Design review of the part built by this model. Coordinates are the model's own, in mm. A direction names the side the tool comes from. Coordinates: 2 decimals unless noted, no trailing zeros. Write each loop counter-clockwise with the first axis right and the second up, starting at its lowest first coordinate (ties: lowest second). Pieces come first, ordered by that corner, then holes. Notation, with made-up numbers: (-33, 30) -> (-28, 30) arc R19 ccw to (-28, 44) -> close; hole circle Ø6 at (15, 76.5). An arc over 180 degrees is marked (long way). Write item = value, one per line. Start each with the question number.
```python
from build123d import *

# Parameters (mm, degrees)
SCHIZZO1_R                     = 3.5
SCHIZZO1_R_2                   = 1.75
ESTRUSIONE_ESTRUSIONE1_DEPTH   = 25
ESTRUSIONE_ESTRUSIONE1_2_DEPTH = 25
ESTRUSIONE_ESTRUSIONE1_3_DEPTH = 25
ESTRUSIONE_ESTRUSIONE1_4_DEPTH = 25
SCHIZZO1_3_R                   = 10.9
SCHIZZO1_3_R_2                 = 5
SCHIZZO1_3_R_3                 = 3
ESTRUSIONE_ESTRUSIONE2_DEPTH   = 3
ESTRUSIONE_ESTRUSIONE4_START   = 3
SCHIZZO1_5_R                   = 10.9
SCHIZZO1_5_R_2                 = 5
ESTRUSIONE_ESTRUSIONE4_DEPTH   = 3
RACCORDO1_R                    = 10


with BuildPart() as part:
    # Schizzo1 → Estrusione-Estrusione1 (new body)
    with BuildSketch(Plane(origin=(0, 0, 0), x_dir=(1, 0, 0), z_dir=(0, 1, 0))):
        with Locations(Location((-15.5, -15.5, 0), (0, 0, 270))):
            Circle(SCHIZZO1_R)
        with Locations(Location((-15.5, -15.5, 0), (0, 0, 270))):
            Circle(SCHIZZO1_R_2, mode=Mode.SUBTRACT)
    extrude(amount=ESTRUSIONE_ESTRUSIONE1_DEPTH)



with BuildPart() as body_2:
    # Schizzo1 → Estrusione-Estrusione1 2 (new body)
    with BuildSketch(Plane(origin=(0, 0, 0), x_dir=(1, 0, 0), z_dir=(0, 1, 0))):
        with Locations(Location((-15.5, 15.5, 0), (0, 0, 270))):
            Circle(SCHIZZO1_R)
        with Locations(Location((-15.5, 15.5, 0), (0, 0, 270))):
            Circle(SCHIZZO1_R_2, mode=Mode.SUBTRACT)
    extrude(amount=ESTRUSIONE_ESTRUSIONE1_2_DEPTH)


with BuildPart() as body_3:
    # Schizzo1 → Estrusione-Estrusione1 3 (new body)
    with BuildSketch(Plane(origin=(0, 0, 0), x_dir=(1, 0, 0), z_dir=(0, 1, 0))):
        with Locations(Location((15.5, 15.5, 0), (0, 0, 270))):
            Circle(SCHIZZO1_R)
        with Locations(Location((15.5, 15.5, 0), (0, 0, 270))):
            Circle(SCHIZZO1_R_2, mode=Mode.SUBTRACT)
    extrude(amount=ESTRUSIONE_ESTRUSIONE1_3_DEPTH)


with BuildPart() as body_4:
    # Schizzo1 → Estrusione-Estrusione1 4 (new body)
    with BuildSketch(Plane(origin=(0, 0, 0), x_dir=(1, 0, 0), z_dir=(0, 1, 0))):
        with Locations(Location((15.5, -15.5, 0), (0, 0, 270))):
            Circle(SCHIZZO1_R)
        with Locations(Location((15.5, -15.5, 0), (0, 0, 270))):
            Circle(SCHIZZO1_R_2, mode=Mode.SUBTRACT)
    extrude(amount=ESTRUSIONE_ESTRUSIONE1_4_DEPTH)


with BuildPart() as part_1:
    add(part.part)

    add(body_2.part)  # Estrusione-Estrusione2 merges body 2

    add(body_3.part)  # Estrusione-Estrusione2 merges body 3

    add(body_4.part)  # Estrusione-Estrusione2 merges body 4
    # Schizzo1<3> → Estrusione-Estrusione2 (add)
    # profile 1 of 6: a face of its own
    with BuildSketch(Plane(origin=(0, 0, 0), x_dir=(1, 0, 0), z_dir=(0, 1, 0))):
        with BuildLine():
            Line((-10.9, 0), (-15.5, -12))
            ThreePointArc((-15.5, -12), (-13.025126266, -13.025126266), (-12, -15.5))
            Line((-12, -15.5), (0, -10.9))
            ThreePointArc((0, -10.9), (-7.707463915, -7.707463915), (-10.9, 0))
        make_face()
    # profile 2 of 6: a face of its own
    with BuildSketch(Plane(origin=(0, 0, 0), x_dir=(1, 0, 0), z_dir=(0, 1, 0))):
        with BuildLine():
            ThreePointArc((10.9, 0), (7.707463915, -7.707463915), (0, -10.9))
            Line((0, -10.9), (12, -15.5))
            ThreePointArc((12, -15.5), (13.025126266, -13.025126266), (15.5, -12))
            Line((15.5, -12), (10.9, 0))
        make_face()
    # profile 3 of 6: a face of its own
    with BuildSketch(Plane(origin=(0, 0, 0), x_dir=(1, 0, 0), z_dir=(0, 1, 0))):
        with BuildLine():
            Line((12, 15.5), (0, 10.9))
            ThreePointArc((0, 10.9), (7.707463915, 7.707463915), (10.9, 0))
            Line((10.9, 0), (15.5, 12))
            ThreePointArc((15.5, 12), (13.025126266, 13.025126266), (12, 15.5))
        make_face()
    # profile 4 of 6: a face of its own
    with BuildSketch(Plane(origin=(0, 0, 0), x_dir=(1, 0, 0), z_dir=(0, 1, 0))):
        with BuildLine():
            Line((-15.5, 12), (-10.9, 0))
            ThreePointArc((-10.9, 0), (-7.707463915, 7.707463915), (0, 10.9))
            Line((0, 10.9), (-12, 15.5))
            ThreePointArc((-12, 15.5), (-13.025126266, 13.025126266), (-15.5, 12))
        make_face()
    # profile 5 of 6: a face of its own
    with BuildSketch(Plane(origin=(0, 0, 0), x_dir=(1, 0, 0), z_dir=(0, 1, 0))):
        Circle(SCHIZZO1_3_R)
        Circle(SCHIZZO1_3_R_2, mode=Mode.SUBTRACT)
    # profile 6 of 6: a face of its own
    with BuildSketch(Plane(origin=(0, 0, 0), x_dir=(1, 0, 0), z_dir=(0, 1, 0))):
        Circle(SCHIZZO1_3_R_2)
        with Locations(Location((0, 0, 0), (0, 0, 270))):
            Circle(SCHIZZO1_3_R_3, mode=Mode.SUBTRACT)
    extrude(amount=ESTRUSIONE_ESTRUSIONE2_DEPTH)

    # Schizzo1<5> → Estrusione-Estrusione4 (add)
    # profile 1 of 5: a face of its own
    with BuildSketch(Plane(origin=(0, 0, 0), x_dir=(1, 0, 0), z_dir=(0, 1, 0)).offset(ESTRUSIONE_ESTRUSIONE4_START)):
        Circle(SCHIZZO1_5_R)
        with Locations(Location((0, 0, 0), (0, 0, 270))):
            Circle(SCHIZZO1_5_R_2, mode=Mode.SUBTRACT)
    # profile 2 of 5: a face of its own
    with BuildSketch(Plane(origin=(0, 0, 0), x_dir=(1, 0, 0), z_dir=(0, 1, 0)).offset(ESTRUSIONE_ESTRUSIONE4_START)):
        with BuildLine():
            Line((-10.9, 0), (-15.5, -12))
            ThreePointArc((-15.5, -12), (-13.025126266, -13.025126266), (-12, -15.5))
            Line((-12, -15.5), (0, -10.9))
            ThreePointArc((0, -10.9), (-7.707463915, -7.707463915), (-10.9, 0))
        make_face()
    # profile 3 of 5: a face of its own
    with BuildSketch(Plane(origin=(0, 0, 0), x_dir=(1, 0, 0), z_dir=(0, 1, 0)).offset(ESTRUSIONE_ESTRUSIONE4_START)):
        with BuildLine():
            Line((-15.5, 12), (-10.9, 0))
            ThreePointArc((-10.9, 0), (-7.707463915, 7.707463915), (0, 10.9))
            Line((0, 10.9), (-12, 15.5))
            ThreePointArc((-12, 15.5), (-13.025126266, 13.025126266), (-15.5, 12))
        make_face()
    # profile 4 of 5: a face of its own
    with BuildSketch(Plane(origin=(0, 0, 0), x_dir=(1, 0, 0), z_dir=(0, 1, 0)).offset(ESTRUSIONE_ESTRUSIONE4_START)):
        with BuildLine():
            Line((12, 15.5), (0, 10.9))
            ThreePointArc((0, 10.9), (7.707463915, 7.707463915), (10.9, 0))
            Line((10.9, 0), (15.5, 12))
            ThreePointArc((15.5, 12), (13.025126266, 13.025126266), (12, 15.5))
        make_face()
    # profile 5 of 5: a face of its own
    with BuildSketch(Plane(origin=(0, 0, 0), x_dir=(1, 0, 0), z_dir=(0, 1, 0)).offset(ESTRUSIONE_ESTRUSIONE4_START)):
        with BuildLine():
            ThreePointArc((10.9, 0), (7.707463915, -7.707463915), (0, -10.9))
            Line((0, -10.9), (12, -15.5))
            ThreePointArc((12, -15.5), (13.025126266, -13.025126266), (15.5, -12))
            Line((15.5, -12), (10.9, 0))
        make_face()
    extrude(amount=ESTRUSIONE_ESTRUSIONE4_DEPTH)

    # Raccordo1
    # the kernel refuses this fillet: 10 mm, written as the material it adds along each edge
    with BuildSketch(Plane(origin=(-15.5, 0, 12), x_dir=(0.3579360116324522, 0, -0.9337461173020496), z_dir=(0, 1, 0)), Plane(origin=(15.5, 0, -12), x_dir=(-0.35793601163245214, 0, 0.9337461173020496), z_dir=(0, 1, 0)), Plane(origin=(-12, 0, -15.5), x_dir=(0.9337461173020497, 0, 0.35793601163245176), z_dir=(0, 1, 0))) as raccordo1_piece_1:
        with BuildLine():
            CenterArc((4.190107638, 10), RACCORDO1_R, 236.464010446, 33.535989554)
            ThreePointArc((-1.334499065, 1.66461034), (-0.537321341, 0.936467115), (0, 0))
            Line((0, 0), (4.190107638, 0))
        make_face()
    extrude(amount=6)
    with BuildSketch(Plane(origin=(-12, 0, 15.5), x_dir=(-0.3047854828813613, 0, 0.952421025295418), z_dir=(0, 1, 0)), Plane(origin=(12, 6, 15.5), x_dir=(0.30478548288135804, 0, 0.9524210252954193), z_dir=(0, -1, 0)), Plane(origin=(15.5, 0, 12), x_dir=(0.9524210252954187, 0, 0.3047854828813593), z_dir=(0, 1, 0)), Plane(origin=(12, 0, -15.5), x_dir=(0.30478548288136037, 0, -0.9524210252954185), z_dir=(0, 1, 0)), Plane(origin=(-15.5, 0, -12), x_dir=(-0.952421025295419, 0, -0.304785482881358), z_dir=(0, 1, 0))) as raccordo1_piece_2:
        with BuildLine():
            CenterArc((5.181353209, 9.524210253), RACCORDO1_R, 218.718751934, 33.535989554)
            Line((-2.620904134, 3.269229809), (0, 0))
            ThreePointArc((0, 0), (1.06674919, 0.166526411), (2.13349838, 0))
        make_face()
    extrude(amount=6)
    with BuildSketch(Plane(origin=(0, 6, 10.9), x_dir=(-0.9337461173020492, 0, 0.3579360116324534), z_dir=(0, -1, 0))) as raccordo1_piece_3:
        with BuildLine():
            CenterArc((RACCORDO1_R * 0.383333333333, -RACCORDO1_R), RACCORDO1_R, 90, 41.946986843)
            Line((-RACCORDO1_R * 0.285109388875, -RACCORDO1_R * 0.256236376847), (0, 0))
            Line((0, 0), (RACCORDO1_R * 0.383333333333, 0))
        make_face()
    extrude(amount=6)
    with BuildSketch(Plane(origin=(10.9, 0, 0), x_dir=(0.35793601163245314, 0, 0.9337461173020493), z_dir=(0, 1, 0)), Plane(origin=(0, 0, -10.9), x_dir=(0.9337461173020492, 0, -0.3579360116324533), z_dir=(0, 1, 0)), Plane(origin=(-10.9, 0, 0), x_dir=(-0.3579360116324529, 0, -0.9337461173020494), z_dir=(0, 1, 0))) as raccordo1_piece_4:
        with BuildLine():
            CenterArc((RACCORDO1_R * 0.383333333333, RACCORDO1_R), RACCORDO1_R, 228.053013157, 41.946986843)
            Line((-RACCORDO1_R * 0.285109388875, RACCORDO1_R * 0.256236376847), (0, 0))
            Line((0, 0), (RACCORDO1_R * 0.383333333333, 0))
        make_face()
    extrude(amount=6)


solid = part_1.part
```
(1) Take a section at B-B, the plane x = 0. State the section outline as (y, z) points, then the cut area to 3 significant figures.
(2) Take a section at D-D, the plane x = -15.5. State the section outline as (y, z) points, then the cut area to 3 significant figures.
(3) For pin 1 Ø11 at (x, z) = (1.5, -2) entering from +Y, flat-tipped, find the tip position at first contact; note if it passes through.
(4) Take a section at C-C, the plane z = 0. State the section outline as (x, y) points.
(5) For line 1 (X direction, y = 8.75, z = 15.5); line 2 (Z direction, x = -14, y = 13.25), list the stretches that pass through material, from the lowest coordinate up.
(6) Take a section at A-A, the plane y = 13. State the section outline as (x, z) points.
(7) For faces 4 (the face through (-10.597, 2.958, 15.405)), 5 (the face through (3.3, 3, -0.1)), 6 (the face through (13.124, 2.958, -5.802)), list the 3-axis set-ups (+Z, -Z, +X, -X, +Y, -Y) from which the entire face can be reached by the end or side of a thin tool; tool diameter is ignored.
(8) Mouldability with a two-part tool opening along Z and no side actions: class faces 1 (the face through (-15.405, 2.958, -10.597)), 2 (the face through (-4, 0, 2)), 3 (the face through (10.597, 2.958, -15.405)) as pulls with the +Z half, pulls with the -Z half, needs draft (parallel to the pull), parting line crosses it, or undercut.
Report:
q1.outline = (0, -11.61) -> (6, -11.61) -> (6, -5) -> (3, -5) -> (3, -3) -> (0, -3) -> close; (0, 3) -> (3, 3) -> (3, 5) -> (6, 5) -> (6, 11.61) -> (0, 11.61) -> close
q1.area = 91.3 mm2
q2.outline = (0, -19) -> (25, -19) -> (25, -17.25) -> (0, -17.25) -> close; (0, -13.75) -> (25, -13.75) -> (25, -12) -> (6, -12) -> (6, -10.72) -> (0, -10.72) -> close; (0, 10.72) -> (6, 10.72) -> (6, 12) -> (25, 12) -> (25, 13.75) -> (0, 13.75) -> close; (0, 17.25) -> (25, 17.25) -> (25, 19) -> (0, 19) -> close
q2.area = 190 mm2
q3.pin_1 = 6
q4.outline = (-11.61, 0) -> (-3, 0) -> (-3, 3) -> (-5, 3) -> (-5, 6) -> (-11.61, 6) -> close; (3, 0) -> (11.61, 0) -> (11.61, 6) -> (5, 6) -> (5, 3) -> (3, 3) -> close
q5.line_1 = -19 to -17.25, -13.75 to -12, 12 to 13.75, 17.25 to 19
q5.line_2 = -18.66 to -16.4, -14.6 to -12.34, 12.34 to 14.6, 16.4 to 18.66
q6.outline = circle Ø7 at (-15.5, -15.5); circle Ø7 at (-15.5, 15.5); circle Ø7 at (15.5, -15.5); circle Ø7 at (15.5, 15.5); hole circle Ø3.5 at (-15.5, -15.5); hole circle Ø3.5 at (-15.5, 15.5); hole circle Ø3.5 at (15.5, -15.5); hole circle Ø3.5 at (15.5, 15.5)
q7.face_4 = +Z, +Y, -Y
q7.face_5 = +Y
q7.face_6 = +X, +Y, -Y
q8.face_1 = undercut
q8.face_2 = needs draft
q8.face_3 = pulls with the -Z half
